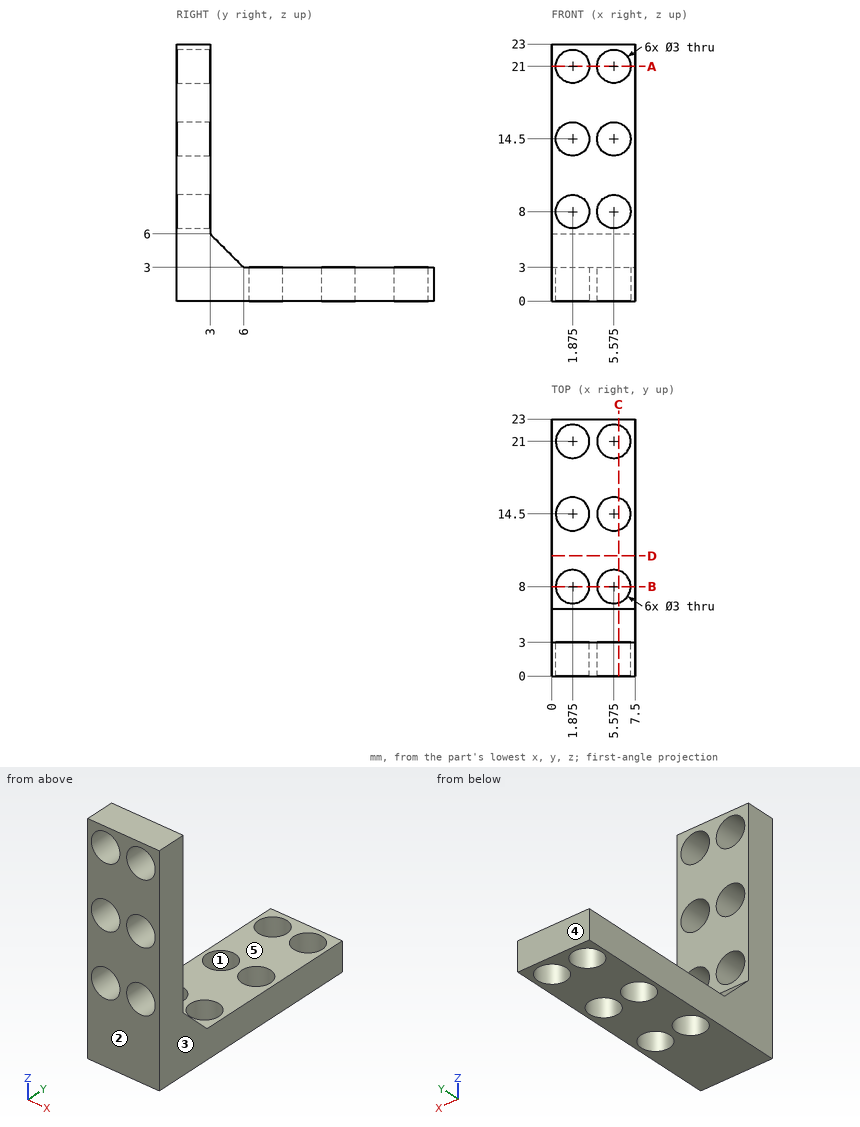
Study the drawing (mm; zero at the part's minimum x, y, z) and answer. A direction names the side the tool comes from. Coordinates: 2 decimals unless noted, no trailing zeros. Write each loop counter-clockwise with the first axis right and the second up, starting at its lowest first coordinate (ties: lowest second). Pieces come first, ordered by that corner, then holes.
Q1. A cutting plane is placed at A-A, the plane z = 21. Give the vertices of the cut face in (x, y) (3 decimals).
Q2. Which of the six approach directions +Z, -Z, +X, -X, +Y, -Y give full straight-line access (tool end or side, diameter ignored) to the marked faces 4 and 5?
Q3. Each of these flat-tipped pins is pushed along its axis until it touches: pin 1 Ø1.8 at (x, z) = (5.575, 21) entering from -Y; pin 2 Ø4 at (x, y) = (4, 11.5) entering from +Z; pin 3 Ø1 at (x, z) = (3, 4.5) entering from +Y; pin 4 Ø4 at (x, z) = (5.5, 14) entering from +Y. Where does it stop, or does it pass through?
Q4. Find the intervals of material crossed by line 1 (X direction, y = 1.8, z = 8) (3 decimals); line 2 (Y direction, x = 5.25, z = 2.5); line 3 (Z direction, x = 0.75, y = 11), in increasing order.
Q5. Determine the mould class of the marked faces 1, 2 and 3 for opening direction X: released by +X, released by -X, zero draft, split by the parting line, or undercut.
Q6. A cutting plane is placed at C-C, the plane x = 6. State how many separate pieces and enclosed holes the cut face has, then the cut area to 3 significant figures.
Q7. A cutting plane is placed at D-D, the plane y = 10.75. Give the vertices of the cut face in (x, z).
Findings below:
1. outline: (0, 0) - (0.375, 0) - (0.375, 3) - (0, 3) - close; (3.375, 0) - (4.075, 0) - (4.075, 3) - (3.375, 3) - close; (7.075, 0) - (7.5, 0) - (7.5, 3) - (7.075, 3) - close
2. face 4: +Z, -Z, +X, -X, +Y
2. face 5: +Z, +X, -X, +Y
3. pin 1: passes through
3. pin 2: stops at z = 3
3. pin 3: stops at y = 5
3. pin 4: stops at y = 3
4. line 1: x = 0 to 0.375, 3.375 to 4.075, 7.075 to 7.5
4. line 2: y = 0 to 6.54, 9.46 to 13.04, 15.96 to 19.54, 22.46 to 23
4. line 3: z = 0 to 3
5. face 1: undercut
5. face 2: zero draft
5. face 3: released by +X
6. separate pieces: 7
6. enclosed holes: 0
6. area: 81.7 mm2
7. outline: (0, 0) - (7.5, 0) - (7.5, 3) - (0, 3) - close
